Can you work these out from the drawing? Everything is in mm from the part's minimum corner. A direction names the side the tool comes from. Round coordinates to 2 decimals unless told otherwise and drop trailing zeros. Order: outer loops, then holes, each group sorted by start corner. A loop starts at its lowest first (then second) coordinate and runs counter-clockwise, first axis right, second up. Notation, with made-up numbers: M -33,11 L -19,11 A29 ccw -19,46 Z; hole C -9,-3 d4. An arc over 180 degrees is marked long. Write item = value, one per line. Start each with the question number.
Item 1: I want a section at C-C, the plane y = 28. List the corners of the cut face in (x, z) for me.
Item 2: I'm going to push flat-ended pins straight in: P1, Ø2, axis at y = 13, z = 9.5, coming from the +X side; P2, Ø1, axis at x = 7, z = 6, coming from the -Y side; P3, Ø8, axis at y = 23, z = 3, coming from the +X side. Where does each tip first touch, or does it pass through?
Item 3: I want a section at B-B, the plane z = 7.5. List the corners of the cut face in (x, y) for me, plus the area to 3 significant figures.
Item 4: Please list where these lines run through material, in increasing order: L1, parallel to Y at x = 11.75, z = 11.25; L2, parallel to Y at x = 10, z = 7.5; L3, parallel to Z at x = 7.5, y = 8.5.
Item 5: I want a section at A-A, the plane x = 7.5. List the corners of the cut face in (y, z) for me.
Item 6: For the marked faces 1 and 2, which set-ups out of +Z, -Z, +X, -X, +Y, -Y let a thin tool reach every point of the face, with its end or its side?
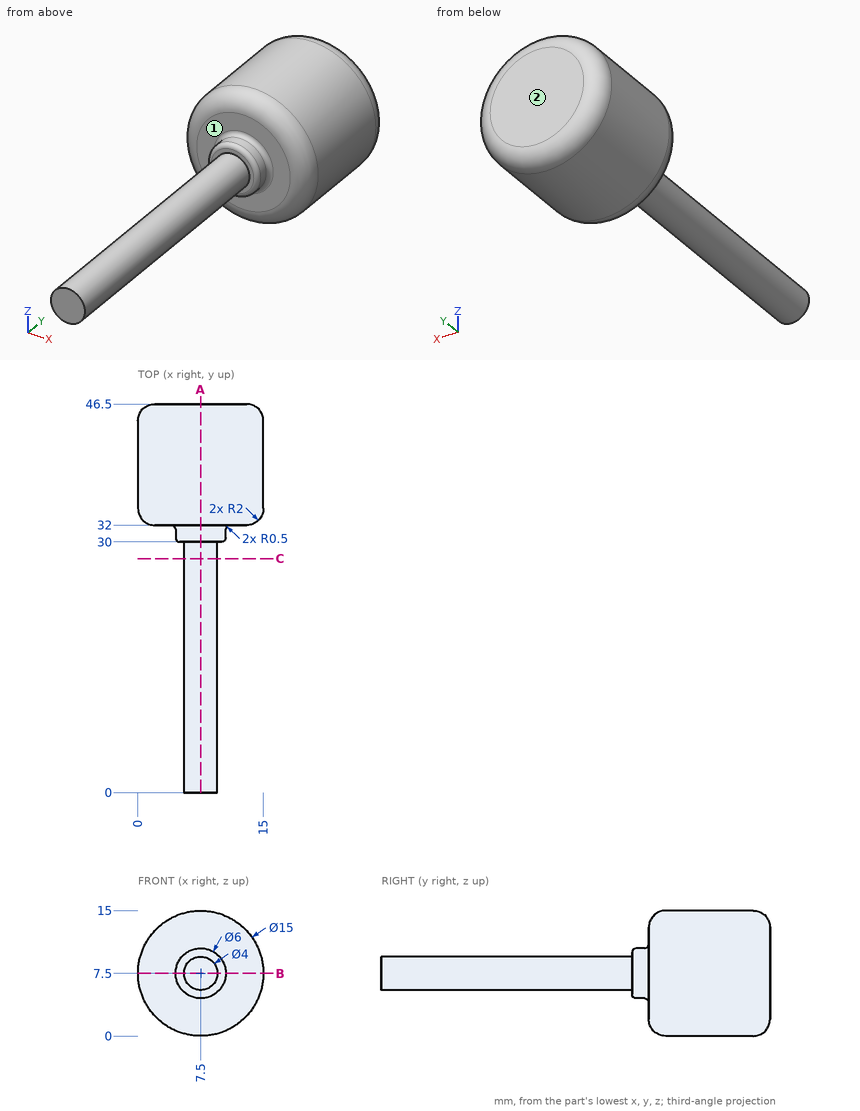
Filled in:
q1.outline = C 7.5,7.5 d4
q2.P1 = 9.23
q2.P2 = 0
q2.P3 = 9.44
q3.outline = M 0,34 A2 ccw 2,32 L 4,32 A0.5 cw 4.5,31.5 L 4.5,30.5 A0.5 ccw 5,30 L 5.5,30 L 5.5,0 L 9.5,0 L 9.5,30 L 10,30 A0.5 ccw 10.5,30.5 L 10.5,31.5 A0.5 cw 11,32 L 13,32 A2 ccw 15,34 L 15,44.5 A2 ccw 13,46.5 L 2,46.5 A2 ccw 0,44.5 Z
q3.area = 346 mm^2
q4.L1 = 32.01 to 46.49
q4.L2 = 30 to 46.5
q4.L3 = 5.5 to 9.5
q5.outline = M 0,5.5 L 30,5.5 L 30,5 A0.5 ccw 30.5,4.5 L 31.5,4.5 A0.5 cw 32,4 L 32,2 A2 ccw 34,0 L 44.5,0 A2 ccw 46.5,2 L 46.5,13 A2 ccw 44.5,15 L 34,15 A2 ccw 32,13 L 32,11 A0.5 cw 31.5,10.5 L 30.5,10.5 A0.5 ccw 30,10 L 30,9.5 L 0,9.5 Z
q6.face_1 = -Y
q6.face_2 = +Z, -Z, +X, -X, +Y
